from build123d import *

# Parameters (mm, degrees)
F1_DEPTH = 32.5
F2_W     = 11
F2_H     = 45
F3_DEPTH = 15.5
F5_DEPTH = 3
F6_SIZE  = 8


with BuildPart() as f1:
    # F0 (on Front) → F1 (new body, symmetric)
    with BuildSketch(Plane.XZ):
        Polygon((8, 0), (0, 0), (0, -3), (11, -3), (11, 15.5), (0, 15.5), (0, 12.5), (8, 12.5), align=None)
    extrude(amount=F1_DEPTH, both=True)

    # F2 (on face) → F3 (cut, through all)
    with BuildSketch(Plane.XY.offset(15.5)):
        with Locations((5.5, 0)):
            Rectangle(F2_W, F2_H)
    extrude(amount=-F3_DEPTH, mode=Mode.SUBTRACT)

    # F4 (on face) → F5 (join, through all)
    with BuildSketch(Plane(origin=(0, 0, -3), x_dir=(1, 0, 0), z_dir=(0, 0, -1))):
        Polygon((11, 22.5), (11, -22.5), (11, -32.5), (26, -32.5), (26, 32.5), (11, 32.5), align=None)
    extrude(amount=-F5_DEPTH)

    # F6
    f6_edges = [f1.edges().sort_by_distance(p)[0] for p in [
        (26, -32.5, -1.5),
        (26, 32.5, -1.5),
    ]]
    chamfer(f6_edges, length=F6_SIZE)


solid = f1.part
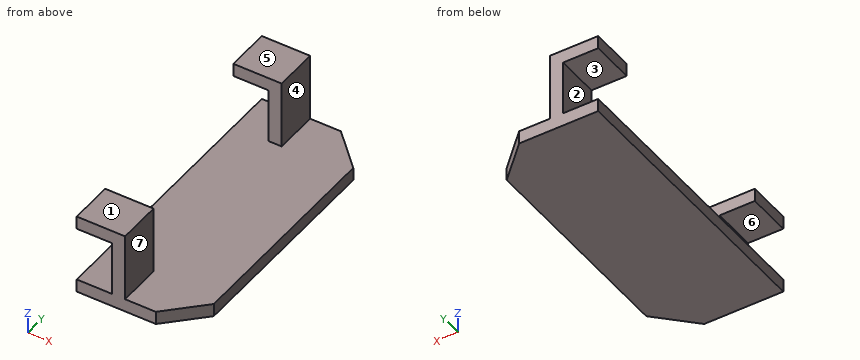
Geometry check sheet. Reference: the model listing, model coordinates, mm. Face numbers are marked on the shaded views. A direction names the side the tool comes from. Give positions to 0.01 mm unless a question says otherwise; leave off trailing zeros. Write each loop counter-clockwise with the first axis right and the second up, starting at its lowest first coordinate (ties: lowest second). Pieces come first, ordered by that corner, then holes. Notation, with made-up numbers: (-21.5, 27) - (15.5, 27) arc R24 ccw to (15.5, 45) - close; hole circle Ø5 at (-24.5, 50). An arc over 180 degrees is marked (long way). Put each result on its own line as item: value.
1. Sectioned sample at B-B, the plane z = 2.5. Enter the section's corners in (x, y).
Ans:
outline: (8, -32.5) - (11, -32.5) - (11, -22.5) - (8, -22.5) - close; (8, 22.5) - (11, 22.5) - (11, 32.5) - (8, 32.5) - close
2. Set-up check for the marked faces 5, 6 and 7: record each of +Z, -Z, +X, -X, +Y, -Y from which the full face is reachable in a straight line by a thin tool's end or side.
Ans:
face 5: +Z, +X, -X, +Y, -Y
face 6: -X, +Y, -Y
face 7: +Z, +X, +Y, -Y
3. Go/stop test with flat-tipped pins: pin 1 (1 mm diameter, centred on x = 11.5, y = -15, fed in from +Z); pin 2 (5 mm diameter, centred on y = 25.5, z = 9.5, fed in from +X); pin 3 (4 mm diameter, centred on y = 14, z = 3.5, fed in from -X); pin 4 (3 mm diameter, centred on y = -25.5, z = 8.5, fed in from -X). Record where each tip stops, or that it passes through.
Ans:
pin 1: stops at z = 0
pin 2: stops at x = 11
pin 3: passes through
pin 4: stops at x = 8
4. Sectioned sample at D-D, the plane x = 16. Enter the section's corners in (y, z), plus the area to 3 significant figures.
Ans:
outline: (-32.5, -3) - (32.5, -3) - (32.5, 0) - (-32.5, 0) - close
area: 195 mm²
5. Sectioned sample at A-A, the plane x = 2.25. Enter the section's corners in (y, z).
Ans:
outline: (-32.5, -3) - (32.5, -3) - (32.5, 0) - (-32.5, 0) - close; (-32.5, 12.5) - (-22.5, 12.5) - (-22.5, 15.5) - (-32.5, 15.5) - close; (22.5, 12.5) - (32.5, 12.5) - (32.5, 15.5) - (22.5, 15.5) - close
6. Sectioned sample at C-C, the plane y = -26.5. Enter the section's corners in (x, z), plus the area to 4 significant figures.
Ans:
outline: (0, -3) - (24, -3) - (24, 0) - (11, 0) - (11, 15.5) - (0, 15.5) - (0, 12.5) - (8, 12.5) - (8, 0) - (0, 0) - close
area: 142.5 mm²
7. Thickness scan on line 1 (Z direction, x = 5.5, y = -27); line 2 (Z direction, x = 16.75, y = -10); line 3 (Y direction, x = 3.5, z = 14.75). Record the ranges inside material, lowest first.
Ans:
line 1: z = -3 to 0, 12.5 to 15.5
line 2: z = -3 to 0
line 3: y = -32.5 to -22.5, 22.5 to 32.5
8. Draft check along Z on the marked faces 1, 2, 3 and 4. Enter one of: +Z half, -Z half, draft (parallel to the pull), parting line (faces both ways), or undercut.
Ans:
face 1: +Z half
face 2: undercut
face 3: undercut
face 4: draft
